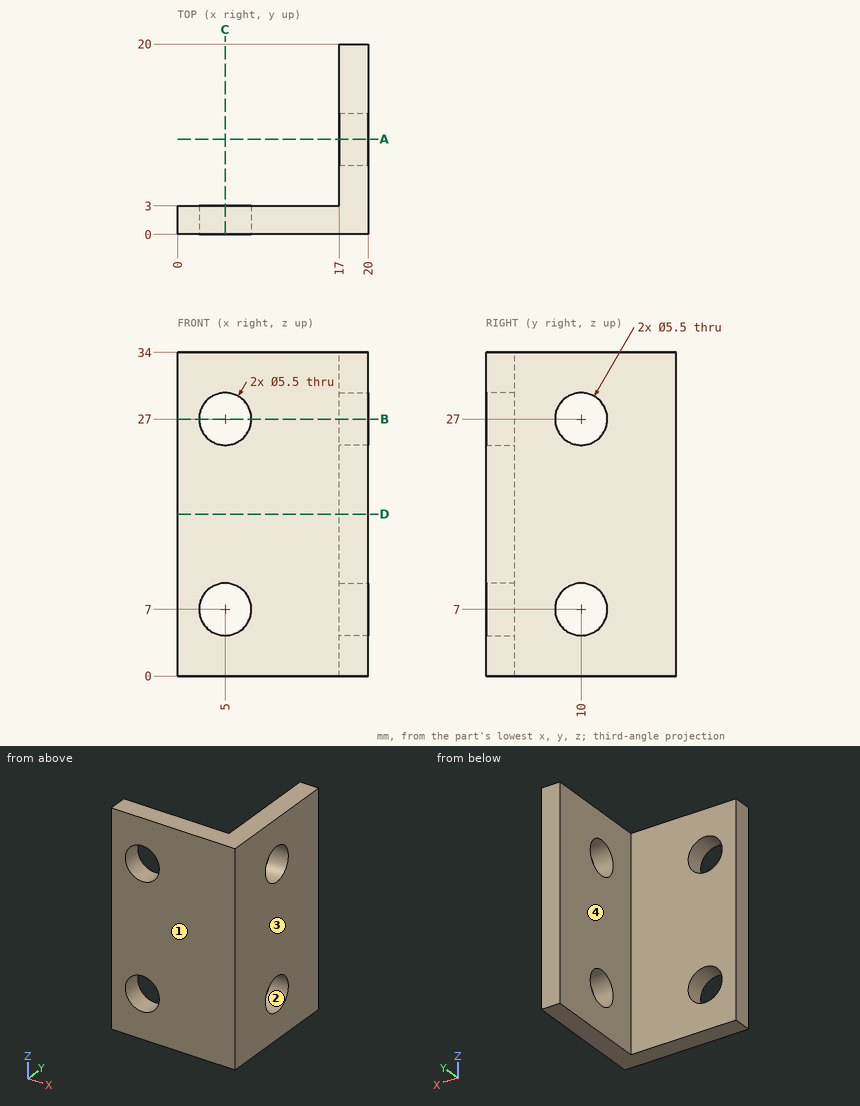
Print and shaded views of the part. All mm, measured from the part's lowest x, y and z. A direction names the side the tool comes from. Coordinates: 2 decimals unless noted, no trailing zeros. Order: outer loops, then holes, each group sorted by start corner. A loop starts at its lowest first (then second) coordinate and runs counter-clockwise, first axis right, second up.
(1) Slice it at D-D, the plane z = 17. Write the cut outline in (x, y), and give its area (3 significant figures).
Check sheet entries:
outline: (0, 0) - (20, 0) - (20, 20) - (17, 20) - (17, 3) - (0, 3) - close
area: 111 mm2
(2) Slice it at A-A, the plane y = 10. Write the cut outline in (x, z), and give its area (3 significant figures).
Check sheet entries:
outline: (17, 0) - (20, 0) - (20, 4.25) - (17, 4.25) - close; (17, 9.75) - (20, 9.75) - (20, 24.25) - (17, 24.25) - close; (17, 29.75) - (20, 29.75) - (20, 34) - (17, 34) - close
area: 69.0 mm2
(3) Slice it at C-C, the plane x = 5. Write the cut outline in (y, z).
Check sheet entries:
outline: (0, 0) - (3, 0) - (3, 4.25) - (0, 4.25) - close; (0, 9.75) - (3, 9.75) - (3, 24.25) - (0, 24.25) - close; (0, 29.75) - (3, 29.75) - (3, 34) - (0, 34) - close
(4) Slice it at B-B, the plane z = 27. Write the cut outline in (x, y), and give its area (3 significant figures).
Check sheet entries:
outline: (0, 0) - (2.25, 0) - (2.25, 3) - (0, 3) - close; (7.75, 0) - (20, 0) - (20, 7.25) - (17, 7.25) - (17, 3) - (7.75, 3) - close; (17, 12.75) - (20, 12.75) - (20, 20) - (17, 20) - close
area: 78.0 mm2
(5) Probe L1, parallel to Y at x = 17.7, z = 7; L2, parallel to X at y = 1.65, z = 27; L3, parallel to Y at x = 6.25, z = 1.5. List the from-to ranges inside material, lowest first.
Check sheet entries:
L1: y = 0 to 7.25, 12.75 to 20
L2: x = 0 to 2.25, 7.75 to 20
L3: y = 0 to 3
(6) Tool access for the marked faces 3 and 4: list every direction of +Z, -Z, +X, -X, +Y, -Y with a clear straight run to the whole face (end or side of a thin tool).
Check sheet entries:
face 3: +Z, -Z, +X, +Y, -Y
face 4: +Z, -Z, -X, +Y
(7) Pin check, flat tips, straight feed: pin 1 Ø3.5 at (y, z) = (10, 27) entering from -X; pin 2 Ø2 at (y, z) = (13, 15) entering from -X; pin 3 Ø1 at (x, z) = (10, 25.5) entering from +Y. Stop position of each tip, or through.
Check sheet entries:
pin 1: passes through
pin 2: stops at x = 17
pin 3: stops at y = 3
(8) Pull direction Z, two halves, no side cores. Call the marked faces 1 and 2: pulls with the +Z half, pulls with the -Z half, needs draft (parallel to the pull), parting line crosses it, or undercut.
Check sheet entries:
face 1: needs draft
face 2: undercut
